```python
from build123d import *

# Parameters (mm, degrees)
CROQUIS1_R                 = 6
SALIENTE_EXTRUIR1_DEPTH    = 76
CORTAR_EXTRUIR1_DEPTH      = 53
CORTAR_EXTRUIR1_DEPTH_BACK = 83
CROQUIS2_W                 = 65
CROQUIS2_H                 = 134.125
CORTAR_EXTRUIR4_DEPTH      = 7
CROQUIS6_R                 = 10.5
CORTAR_EXTRUIR5_DEPTH      = 7


with BuildPart() as part:
    # Croquis1 → Saliente-Extruir1 (new body)
    with BuildSketch(Plane.XY):
        with BuildLine():
            Line((3.623560213, 29.985380117), (40.623560213, 29.985380117))
            add(Edge.make_bspline(
                [(40.623560213, 29.985380117), (44.757987914, -45.934087744), (-12.775954516, -106.998983358)],
                knots=[0, 0, 0, 1, 1, 1], degree=2))
            ThreePointArc((-12.775954516, -106.998983358), (-25.787263181, -113.574217266), (-31.882365072, -100.331196951))
            add(Edge.make_bspline(
                [(3.623560213, 29.985380117), (6.510357156, -38.808737065), (-31.882365072, -100.331196951)],
                knots=[0, 0, 0, 1, 1, 1], degree=2))
        make_face()
        with Locations((-22.451139251, -104.014619883)):
            Circle(CROQUIS1_R, mode=Mode.SUBTRACT)
    extrude(amount=SALIENTE_EXTRUIR1_DEPTH)

    # Croquis2 → Cortar-Extruir1 (cut, two sides: drawn at the far end of the back side and taken through both)
    with BuildSketch(Plane(origin=(0, 0, 0), x_dir=(0, 0, -1), z_dir=(1, 0, 0)).offset(-CORTAR_EXTRUIR1_DEPTH_BACK)):
        with Locations((-38, -47.077119883)):
            Rectangle(CROQUIS2_W, CROQUIS2_H)
    extrude(amount=CORTAR_EXTRUIR1_DEPTH + CORTAR_EXTRUIR1_DEPTH_BACK, mode=Mode.SUBTRACT)

    # Croquis5 → Cortar-Extruir4 (cut)
    with BuildSketch(Plane.XZ.offset(-19.985380117)):
        with BuildLine():
            Line((10.825063576, 63.739022161), (33.900709288, 63.739022161))
            ThreePointArc((33.900709288, 63.739022161), (36.729136412, 62.567449286), (37.900709288, 59.739022161))
            Line((37.900709288, 59.739022161), (37.900709288, 11.860366898))
            ThreePointArc((37.900709288, 11.860366898), (36.729136412, 9.031939774), (33.900709288, 7.860366898))
            Line((33.900709288, 7.860366898), (10.825063576, 7.860366898))
            ThreePointArc((10.825063576, 7.860366898), (7.996636452, 9.031939774), (6.825063576, 11.860366898))
            Line((6.825063576, 11.860366898), (6.825063576, 59.739022161))
            ThreePointArc((6.825063576, 59.739022161), (7.996636452, 62.567449286), (10.825063576, 63.739022161))
        make_face()
    extrude(amount=-CORTAR_EXTRUIR4_DEPTH, mode=Mode.SUBTRACT)

    # Croquis6 → Cortar-Extruir5 (cut)
    with BuildSketch(Plane(origin=(0, 26.985380117, 0), x_dir=(-1, 0, 0), z_dir=(0, -1, 0))):
        with Locations(Location((-22.362886432, -35.79969453, 0), (0, 0, 90))):
            Circle(CROQUIS6_R)
    extrude(amount=-CORTAR_EXTRUIR5_DEPTH, mode=Mode.SUBTRACT)


solid = part.part
```
For this review, take the finished solid that the model builds, in its own axes (mm). A direction names the side the tool comes from. Coordinates: 2 decimals unless noted, no trailing zeros. Put each result on its own line as item: value.
1. Mouldability with a two-part tool opening along Z and no side actions: class faces 1 (the cylindrical face through (-25.571, -113.647, 73.212)), 2 (the flat face through (9, -36, 76)), 3 (the cylindrical face through (7.97, 23.44, 62.54)) as released by +Z, released by -Z, zero draft, split by the parting line, or undercut.
Values found:
face 1: zero draft
face 2: released by +Z
face 3: undercut
2. Wall thickness on probe 1 along Z at (x, y) = (3.5, -55); probe 2 along Y at (x, z) = (7.5, 49.5); probe 3 along Y at (x, z) = (6.5, 25.5): over which ranges is each line inside the solid? List them lowest first.
Values found:
probe 1: 0 to 5.5, 70.5 to 76
probe 2: 26.99 to 29.99
probe 3: 19.99 to 29.99
3. For pin 1 (11 mm diameter, centred on x = 28, z = 52.5, fed in from -Y); pin 2 (12.5 mm diameter, centred on x = 22.36, z = 35.8, fed in from -Y); pin 3 (4 mm diameter, centred on x = 26, z = 64.5, fed in from -Y), all flat-tipped, find the tip position at first contact; note any pin that passes through.
Values found:
pin 1: y = 26.99
pin 2: through
pin 3: y = 19.99
4. Add section A-A, the plane x = -18. Count the separate pieces of the cut face and the enclosed holes in it, then the cut area to 3 significant figures.
Values found:
separate pieces: 4
enclosed holes: 0
area: 330 mm²
5. Machinability: for faces 4 (the flat face through (12, -33, 5.5)), 5 (the flat face through (9, -36, 0)), 6 (the flat face through (6.825, 23, 35)), which of the approach directions +Z, -Z, +X, -X, +Y, -Y give a long, thin tool a straight path to every point of the face, cutting with its end or side? Answer none if there is none.
Values found:
face 4: +X, -X, -Y
face 5: -Z, +X, -X, +Y, -Y
face 6: -Y
